Geometry check sheet. Reference: drawing and pictorial views, mm from the part's lowest x, y, z. Coordinates: 2 decimals unless noted, no trailing zeros. Write each loop counter-clockwise with the first axis right and the second up, starting at its lowest first coordinate (ties: lowest second). Pieces come first, ordered by that corner, then holes. Notation, with made-up numbers: (-26.75, -34.5) -> (29.25, -34.5) arc R15 cw to (29.25, -5.5) -> close; hole circle Ø9 at (-22.5, 62). An arc over 180 degrees is marked (long way). Use a Markdown table: item, result. Add a question column.
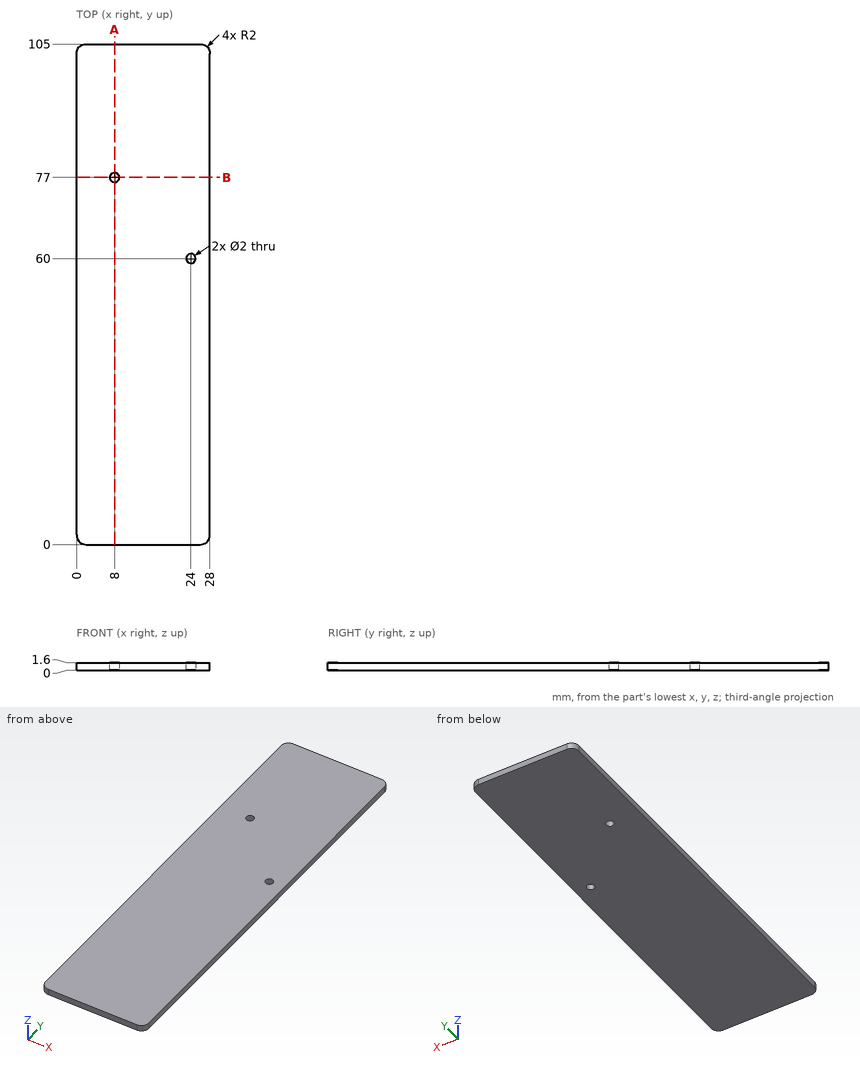
1) Thickness scan on L1, parallel to X at y = 60, z = 0.6; L2, parallel to Y at x = 8, z = 1.1; L3, parallel to Y at x = 24, z = 1.2. Record the ranges inside material, lowest first.
2) Cross-section at A-A on x = 8. Record the boundary of the cut face in (y, z).
3) Cross-section at B-B on y = 77. Record the boundary of the cut face in (x, z).
4) Gauge pin test, flat end, axial feed: pin 1 (1.6 mm diameter, centred on x = 8, y = 77, fed in from -Z). Record the tip position at first contact, or that the pin passes through.
Returned:
| question | item | result |
|---|---|---|
| 1 | L1 | x = 0 to 23, 25 to 28 |
| 1 | L2 | y = 0 to 76, 78 to 105 |
| 1 | L3 | y = 0 to 59, 61 to 105 |
| 2 | outline | (0, 0) -> (76, 0) -> (76, 1.6) -> (0, 1.6) -> close; (78, 0) -> (105, 0) -> (105, 1.6) -> (78, 1.6) -> close |
| 3 | outline | (0, 0) -> (7, 0) -> (7, 1.6) -> (0, 1.6) -> close; (9, 0) -> (28, 0) -> (28, 1.6) -> (9, 1.6) -> close |
| 4 | pin 1 | passes through |
